from build123d import *

# Parameters (mm, degrees)
BOSS_EXTRUDE1_DEPTH                            = 3
BOSS_EXTRUDE2_DEPTH                            = 15
SKETCH4_W                                      = 13
SKETCH4_H                                      = 3
BOSS_EXTRUDE3_DEPTH                            = 12
BOSS_EXTRUDE4_DEPTH                            = 3
BOSS_EXTRUDE5_DEPTH                            = 3
SKETCH7_R                                      = 1.525
BOSS_EXTRUDE6_DEPTH                            = 3
BOSS_EXTRUDE7_START                            = 3
SKETCH8_R                                      = 1.525
BOSS_EXTRUDE7_DEPTH                            = 3
BOSS_EXTRUDE8_DEPTH                            = 3
FILLET2_R                                      = 10
FILLET3_R                                      = 5
CSK_START                                      = -8
CSK_SLOT_FOR_M3_FLAT_HEAD_MACHINE_SCREW1_DEPTH = 3
F_3_0MM_DOWEL_HOLE2_D                          = 3
F_3_0MM_DOWEL_HOLE2_DEPTH                      = 7.5
F_3_0MM_DOWEL_HOLE2_CSINK_D                    = 3.05
F_3_0MM_DOWEL_HOLE2_CSINK_ANGLE                = 90
F_3_0MM_DOWEL_HOLE2_TIP                        = 0.901290929


with BuildPart() as part:
    # Sketch1 → Boss-Extrude1 (new body)
    with BuildSketch(Plane.XY):
        Polygon((139, -5), (109.876604516, -5), (74.70251528, -19.102143128), (40.663008058, -5), (11, -5), (11, -59.019998994), (139, -59.019998994), align=None)
        Polygon((126, -11.464259225), (90.561608439, -25.672367549), (126, -40.354051004), align=None, mode=Mode.SUBTRACT)
        Polygon((24, -11.085769738), (24, -39.430007843), (58.769174389, -25.49020487), align=None, mode=Mode.SUBTRACT)
        Polygon((39.809790244, -46.019998994), (108.323633524, -46.019998994), (74.628267548, -32.06042929), align=None, mode=Mode.SUBTRACT)
    extrude(amount=-BOSS_EXTRUDE1_DEPTH)

    # Sketch3 → Boss-Extrude2 (add)
    with BuildSketch(Plane(origin=(0, 0, -3), x_dir=(-1, 0, 0), z_dir=(0, 0, -1))):
        Polygon((-139, -8), (-139, -5), (-126, -5), (-126, -56.019998994), (-24, -56.019998994), (-24, -5), (-11, -5), (-11, -8), (-21, -8), (-21, -59.019998994), (-129, -59.019998994), (-129, -8), align=None)
    extrude(amount=BOSS_EXTRUDE2_DEPTH)

    # Sketch4 → Boss-Extrude3 (add)
    with BuildSketch(Plane(origin=(0, 0, -18), x_dir=(-1, 0, 0), z_dir=(0, 0, -1))):
        with Locations((-132.5, -6.5)):
            Rectangle(SKETCH4_W, SKETCH4_H)
        with Locations((-17.5, -6.5)):
            Rectangle(SKETCH4_W, SKETCH4_H)
    extrude(amount=BOSS_EXTRUDE3_DEPTH)

    # Sketch5 → Boss-Extrude4 (add)
    with BuildSketch(Plane.ZY.offset(-21)):
        Polygon((-30, -8), (-18, -8), (-18, -59.019998994), align=None)
    extrude(amount=-BOSS_EXTRUDE4_DEPTH)

    # Sketch6 → Boss-Extrude5 (add)
    with BuildSketch(Plane(origin=(129, 0, 0), x_dir=(0, 0, -1), z_dir=(1, 0, 0))):
        Polygon((18, -8), (18, -59.019998994), (30, -8), align=None)
    extrude(amount=-BOSS_EXTRUDE5_DEPTH)

    # Sketch7 → Boss-Extrude6 (add)
    with BuildSketch(Plane(origin=(50.603026188, 28.677278628, 20.937913876), x_dir=(0, 0.9992078437352027, -0.039795540177848664), z_dir=(-1, 0, 0))):
        with BuildLine():
            Line((-86.078252358, 42.397029499), (-86.675185461, 27.408911843))
            Line((-86.675185461, 27.408911843), (-86.794572081, 24.411288312))
            Line((-86.794572081, 24.411288312), (-108.590752447, 16.032710832))
            ThreePointArc((-108.590752447, 16.032710832), (-118.903275809, 20.564727028), (-114.461076578, 30.916257103))
            Line((-114.461076578, 30.916257103), (-86.078252358, 42.397029499))
        make_face()
        with Locations(Location((-111.454014111, 23.696060126, 0), (0, 0, 267.719281244))):
            Circle(SKETCH7_R, mode=Mode.SUBTRACT)
    extrude(amount=BOSS_EXTRUDE6_DEPTH)

    # Sketch8 → Boss-Extrude7 (add)
    with BuildSketch(Plane(origin=(100.803026188, 28.677278628, 20.937913876), x_dir=(0, -0.9992078437352027, 0.039795540177848664), z_dir=(1, 0, 0)).offset(BOSS_EXTRUDE7_START)):
        with BuildLine():
            Line((86.078252358, 42.397029499), (86.675185461, 27.408911843))
            Line((86.675185461, 27.408911843), (86.794572081, 24.411288312))
            Line((86.794572081, 24.411288312), (108.590752447, 16.032710832))
            ThreePointArc((108.590752447, 16.032710832), (118.903275809, 20.564727028), (114.461076578, 30.916257103))
            Line((114.461076578, 30.916257103), (86.078252358, 42.397029499))
        make_face()
        with Locations(Location((111.454014111, 23.696060126, 0), (0, 0, 272.280718756))):
            Circle(SKETCH8_R, mode=Mode.SUBTRACT)
    extrude(amount=-BOSS_EXTRUDE7_DEPTH)

    # Sketch9 → Boss-Extrude8 (add)
    with BuildSketch(Plane.XY):
        Polygon((11, -59.019998994), (47.603026188, -59.019998994), (47.603026188, -80.465483362), align=None)
        Polygon((103.803026188, -59.019998994), (139, -59.019998994), (103.803026188, -80.465483362), align=None)
    extrude(amount=-BOSS_EXTRUDE8_DEPTH)

    # Fillet2
    fillet2_edges = [part.edges().sort_by_distance(p)[0] for p in [
        (50.603026188, -59.019998994, -9),
        (103.803026188, -59.019998994, -10.5),
        (100.803026188, -59.019998994, -9),
        (47.603026188, -59.019998994, -10.5),
    ]]
    fillet(fillet2_edges, radius=FILLET2_R)

    # Fillet3
    fillet3_edges = [part.edges().sort_by_distance(p)[0] for p in [
        (47.603026188, -69.742741178, 0),
        (29.301513094, -59.019998994, -3),
        (103.803026188, -69.742741178, 0),
        (103.803026188, -74.742741178, -3),
        (121.401513094, -59.019998994, -3),
        (106.731958376, -61.948931182, -3),
        (47.603026188, -74.742741178, -3),
        (44.674094, -61.948931182, -3),
    ]]
    fillet(fillet3_edges, radius=FILLET3_R)

    # CSK SLOT for M3 Flat Head Machine Screw1: read off the stored shape, not the designer's step
    # CSK SLOT for M3 Flat Head Machine Sc 2 → CSK SLOT for M3 Flat Head Machine Screw1 (cut)
    with BuildSketch(Plane(origin=(0, 0, 0), x_dir=(1, 0, 0), z_dir=(0, 1, 0)).offset(CSK_START)):
        with BuildLine():
            ThreePointArc((17, 4.3), (18.7, 6), (17, 7.7))
            Line((17, 7.7), (15, 7.7))
            ThreePointArc((15, 7.7), (13.3, 6), (15, 4.3))
            Line((15, 4.3), (17, 4.3))
        make_face()
        with BuildLine():
            ThreePointArc((133, 7.7), (131.3, 6), (133, 4.3))
            Line((133, 4.3), (135, 4.3))
            ThreePointArc((135, 4.3), (136.7, 6), (135, 7.7))
            Line((135, 7.7), (133, 7.7))
        make_face()
    extrude(amount=CSK_SLOT_FOR_M3_FLAT_HEAD_MACHINE_SCREW1_DEPTH, mode=Mode.SUBTRACT)

    # CSK SLOT for M3 Flat Head Machine Sc 3: loft between two sections, ruled curve by curve
    csk_slot_for_m3_flat_head_machine_sc_3_from = [
        Edge.make_three_point_arc((17, -6.55, -7.7), (18.202081528, -6.55, -7.202081528), (18.7, -6.55, -6)),
        Edge.make_three_point_arc((18.7, -6.55, -6), (18.202081528, -6.55, -4.797918472), (17, -6.55, -4.3)),
        Edge.make_three_point_arc((15, -6.55, -4.3), (13.797918472, -6.55, -4.797918472), (13.3, -6.55, -6)),
        Edge.make_three_point_arc((13.3, -6.55, -6), (13.797918472, -6.55, -7.202081528), (15, -6.55, -7.7)),
        Edge.make_line((17, -6.55, -4.3), (15, -6.55, -4.3)),
        Edge.make_line((17, -6.55, -7.7), (15, -6.55, -7.7)),
    ]
    csk_slot_for_m3_flat_head_machine_sc_3_to = [
        Edge.make_three_point_arc((17, -8, -9.15), (19.227386361, -8, -8.227386361), (20.15, -8, -6)),
        Edge.make_three_point_arc((20.15, -8, -6), (19.227386361, -8, -3.772613639), (17, -8, -2.85)),
        Edge.make_three_point_arc((15, -8, -2.85), (12.772613639, -8, -3.772613639), (11.85, -8, -6)),
        Edge.make_three_point_arc((11.85, -8, -6), (12.772613639, -8, -8.227386361), (15, -8, -9.15)),
        Edge.make_line((17, -8, -2.85), (15, -8, -2.85)),
        Edge.make_line((17, -8, -9.15), (15, -8, -9.15)),
    ]
    csk_slot_for_m3_flat_head_machine_sc_3 = Solid(Shell([*[Face.make_surface_from_curves(csk_slot_for_m3_flat_head_machine_sc_3_from[k], csk_slot_for_m3_flat_head_machine_sc_3_to[k]) for k in range(6)], Face(Wire(csk_slot_for_m3_flat_head_machine_sc_3_from)), Face(Wire(csk_slot_for_m3_flat_head_machine_sc_3_to))]))
    add(csk_slot_for_m3_flat_head_machine_sc_3, mode=Mode.SUBTRACT)

    # CSK SLOT for M3 Flat Head Machine Sc 4: loft between two sections, ruled curve by curve
    csk_slot_for_m3_flat_head_machine_sc_4_from = [
        Edge.make_three_point_arc((135, -6.55, -7.7), (136.202081528, -6.55, -7.202081528), (136.7, -6.55, -6)),
        Edge.make_three_point_arc((136.7, -6.55, -6), (136.202081528, -6.55, -4.797918472), (135, -6.55, -4.3)),
        Edge.make_three_point_arc((133, -6.55, -4.3), (131.797918472, -6.55, -4.797918472), (131.3, -6.55, -6)),
        Edge.make_three_point_arc((131.3, -6.55, -6), (131.797918472, -6.55, -7.202081528), (133, -6.55, -7.7)),
        Edge.make_line((135, -6.55, -4.3), (133, -6.55, -4.3)),
        Edge.make_line((135, -6.55, -7.7), (133, -6.55, -7.7)),
    ]
    csk_slot_for_m3_flat_head_machine_sc_4_to = [
        Edge.make_three_point_arc((135, -8, -9.15), (137.227386361, -8, -8.227386361), (138.15, -8, -6)),
        Edge.make_three_point_arc((138.15, -8, -6), (137.227386361, -8, -3.772613639), (135, -8, -2.85)),
        Edge.make_three_point_arc((133, -8, -2.85), (130.772613639, -8, -3.772613639), (129.85, -8, -6)),
        Edge.make_three_point_arc((129.85, -8, -6), (130.772613639, -8, -8.227386361), (133, -8, -9.15)),
        Edge.make_line((135, -8, -2.85), (133, -8, -2.85)),
        Edge.make_line((135, -8, -9.15), (133, -8, -9.15)),
    ]
    csk_slot_for_m3_flat_head_machine_sc_4 = Solid(Shell([*[Face.make_surface_from_curves(csk_slot_for_m3_flat_head_machine_sc_4_from[k], csk_slot_for_m3_flat_head_machine_sc_4_to[k]) for k in range(6)], Face(Wire(csk_slot_for_m3_flat_head_machine_sc_4_from)), Face(Wire(csk_slot_for_m3_flat_head_machine_sc_4_to))]))
    add(csk_slot_for_m3_flat_head_machine_sc_4, mode=Mode.SUBTRACT)

    # Ø3.0mm Dowel Hole2
    with Locations(Plane(origin=(134, -8, -25), x_dir=(0, 0, -1), z_dir=(0, -1, 0))):
        with Locations((0, 0), (0, -118.445937781)):
            CounterSinkHole(F_3_0MM_DOWEL_HOLE2_D / 2, F_3_0MM_DOWEL_HOLE2_CSINK_D / 2, depth=F_3_0MM_DOWEL_HOLE2_DEPTH, counter_sink_angle=F_3_0MM_DOWEL_HOLE2_CSINK_ANGLE)
            with Locations((0, 0, -(F_3_0MM_DOWEL_HOLE2_DEPTH + F_3_0MM_DOWEL_HOLE2_TIP / 2))):  # 118° drill point
                Cone(0, F_3_0MM_DOWEL_HOLE2_D / 2, F_3_0MM_DOWEL_HOLE2_TIP, mode=Mode.SUBTRACT)


solid = part.part
The listing builds one solid part. Answer for the finished solid, in the listing's coordinates (mm). A direction names the side the tool comes from. Coordinates: 2 decimals unless noted, no trailing zeros. Write each loop counter-clockwise with the first axis right and the second up, starting at its lowest first coordinate (ties: lowest second). Pieces come first, ordered by that corner, then holes. Notation, with made-up numbers: M 5.25,60 L 56.25,60 A7 ccw 56.25,65 Z; hole C 74,30.25 d4. An arc over 180 degrees is marked long. Put each result on its own line as item: value. Start each with the question number.
1. Flat-ended cylindrical pins translate along their axes: P1, Ø15, axis at y = -39.5, z = -12.5, coming from the +X side; P2, Ø3, axis at y = -21.5, z = -3.5, coming from the +X side; P3, Ø3, axis at x = 16.5, z = -22, coming from the -Y side; P4, Ø4, axis at x = 72.5, z = -15.5, coming from the -Y side. Find the tip coordinate at first contact, or state that the pin passes through.
2. A cutting plane is placed at D-D on x = 95. Write down the section's boundary in (y, z).
3. A cutting plane is placed at A-A on z = 7. Write down the section's boundary in (x, y).
4. A cutting plane is placed at B-B on x = 63.5. Write down the section's boundary in (y, z).
5. Consider line 1 (Z direction, x = 134, y = -6.3); line 2 (X direction, y = -6.65, z = -25); line 3 (X direction, y = -16, z = -12). Determine where each line is inside the solid, lowest interval first. Write a range as from..to.
6. A cutting plane is placed at C-C on y = -22.5. Write down the section's boundary in (x, z), then the cut area to 3 significant figures.
7. For a pull along X with two mould halves and no side action, classify faces 5 (the flat face through (102.36, -68.9, -13.54)), 6 (the flat face through (126, -32, -15)), 7 (the cylindrical face through (44.751, -62.027, -11.819)) as pulls with the +X half, pulls with the -X half, needs draft (parallel to the pull), parting line crosses it, or undercut.
8. Which of the six approach directions +Z, -Z, +X, -X, +Y, -Y give full straight-line access (tool end or side, diameter ignored) to faces 1 (the flat face through (129, -29, -13)), 2 (the flat face through (20, -43, -3)), 3 (the flat face through (47.603, -83, -2)), 4 (the flat face through (100.803, -80, 1))?
Resolved:
1. P1: stops at x = 129
1. P2: stops at x = 139
1. P3: stops at y = -8
1. P4: stops at y = -59.02
2. outline: M -59.94,-17.58 L -59.02,-18 L -56.02,-18 L -56.02,-3 L -46.02,-3 L -46.02,0 L -59.02,0 L -59.94,0.4 Z; M -40.5,-3 L -27.51,-3 L -27.51,0 L -40.5,0 Z; M -23.89,-3 L -10.96,-3 L -10.96,0 L -23.89,0 Z
3. outline: M 47.6,-89.79 L 50.6,-89.79 L 50.6,-75.27 L 47.6,-75.27 Z; M 100.8,-89.79 L 103.8,-89.79 L 103.8,-75.27 L 100.8,-75.27 Z
4. outline: M -59.02,-18 L -56.02,-18 L -56.02,-3 L -46.02,-3 L -46.02,0 L -59.02,0 Z; M -36.52,-3 L -14.46,-3 L -14.46,0 L -36.52,0 Z
5. line 1: z = -30..-26.5, -23.5..-7.7, -4.3..0
5. line 2: x = 11..14.05, 17.05..24, 126..132.5, 135.5..139
5. line 3: x = 21..24, 126..129
6. outline: M 11,-3 L 21,-3 L 21,-26.59 L 24,-26.59 L 24,0 L 11,0 Z; M 51.55,-3 L 98.47,-3 L 98.47,0 L 51.55,0 Z; M 126,-26.59 L 129,-26.59 L 129,-3 L 139,-3 L 139,0 L 126,0 Z
6. area: 360 mm2
7. face 5: needs draft
7. face 6: undercut
7. face 7: pulls with the -X half
8. face 1: -Z, +X, -Y
8. face 2: -Z, -X, -Y
8. face 3: -X, -Y
8. face 4: +Z, -Z, -Y
